Geometry check sheet. Reference: the model listing, model coordinates, mm. Give positions to 0.01 mm unless a question says otherwise; leave off trailing zeros. Order: outer loops, then holes, each group sorted by start corner. A loop starts at its lowest first (then second) coordinate and runs counter-clockwise, first axis right, second up.
from build123d import *

# Parameters (mm, degrees)
SKETCH1_R           = 1.355900406
BOSS_EXTRUDE1_DEPTH = 1.5875
SKETCH2_R           = 3.175
BOSS_EXTRUDE2_DEPTH = 1.5875
SKETCH3_R           = 1.524
CUT_EXTRUDE1_DEPTH  = 436.184338179
SKETCH5_W           = 2.10299656
SKETCH5_H           = 13.208
BOSS_EXTRUDE3_DEPTH = 1.5875


with BuildPart() as part:
    # Sketch1 → Boss-Extrude1 (new body)
    with BuildSketch(Plane.XY):
        with BuildLine():
            Line((-301.9473, 111.74645), (-305.87795, 115.6771))
            Line((-305.87795, 115.6771), (-316.1078, 115.6771))
            Line((-316.1078, 115.6771), (-316.1078, 128.8851))
            Line((-316.1078, 128.8851), (-305.87795, 128.8851))
            Line((-305.87795, 128.8851), (-301.9473, 132.81575))
            Line((-301.9473, 132.81575), (-301.9473, 150.9704))
            ThreePointArc((-301.9473, 150.9704), (-303.063223164, 153.664476836), (-305.7573, 154.7804))
            Line((-305.7573, 154.7804), (-397.247125, 154.7804))
            ThreePointArc((-397.247125, 154.7804), (-399.946077222, 153.659592612), (-401.0571, 150.956597849))
            Line((-401.0571, 150.956597849), (-401.0571, 148.341))
            Line((-401.0571, 148.341), (-399.1521, 148.341))
            Line((-399.1521, 148.341), (-399.1521, 95.6449))
            Line((-399.1521, 95.6449), (-401.0571, 95.6449))
            Line((-401.0571, 95.6449), (-401.0571, 91.659304166))
            ThreePointArc((-401.0571, 91.659304166), (-399.951018769, 88.947400452), (-397.2472, 87.8217))
            Line((-397.2472, 87.8217), (-378.5565, 87.8217))
            Line((-378.5565, 87.8217), (-368.3165, 91.1883))
            Line((-368.3165, 91.1883), (-315.9973, 91.1883))
            Line((-315.9973, 91.1883), (-305.7573, 87.8217))
            ThreePointArc((-305.7573, 87.8217), (-303.063223164, 88.937623164), (-301.9473, 91.6317))
            Line((-301.9473, 91.6317), (-301.9473, 111.74645))
        make_face()
        with Locations((-305.7573, 91.6317)):
            Circle(SKETCH1_R, mode=Mode.SUBTRACT)
        with Locations((-305.7573, 150.9704)):
            Circle(SKETCH1_R, mode=Mode.SUBTRACT)
        with Locations((-397.247125, 150.9704)):
            Circle(SKETCH1_R, mode=Mode.SUBTRACT)
        with Locations((-397.2472, 91.6317)):
            Circle(SKETCH1_R, mode=Mode.SUBTRACT)
    extrude(amount=BOSS_EXTRUDE1_DEPTH)

    # Sketch2 → Boss-Extrude2 (add)
    # profile 1 of 2: a face of its own
    with BuildSketch(Plane.XY.offset(1.5875)):
        with BuildLine():
            Line((-361.0272, 159.40105), (-361.0272, 154.7804))
            Line((-361.0272, 154.7804), (-341.9772, 154.7804))
            Line((-341.9772, 154.7804), (-341.9772, 159.40105))
            ThreePointArc((-341.9772, 159.40105), (-351.5022, 168.92605), (-361.0272, 159.40105))
        make_face()
        with Locations((-351.5022, 159.40105)):
            Circle(SKETCH2_R, mode=Mode.SUBTRACT)
    # profile 2 of 2: a face of its own
    with BuildSketch(Plane.XY.offset(1.5875)):
        with BuildLine():
            Line((-341.9772, 91.1883), (-361.0272, 91.1883))
            Line((-361.0272, 91.1883), (-361.0272, 83.20105))
            ThreePointArc((-361.0272, 83.20105), (-351.5022, 73.67605), (-341.9772, 83.20105))
            Line((-341.9772, 83.20105), (-341.9772, 91.1883))
        make_face()
        with Locations((-351.5022, 83.20105)):
            Circle(SKETCH2_R, mode=Mode.SUBTRACT)
    extrude(amount=-BOSS_EXTRUDE2_DEPTH)

    # Sketch3 → Cut-Extrude1 (cut, through all)
    with BuildSketch(Plane.XY.offset(1.5875)):
        with Locations((-397.247125, 150.9704)):
            Circle(SKETCH3_R)
        with Locations((-305.7573, 150.9704)):
            Circle(SKETCH3_R)
        with Locations((-305.7573, 91.6317)):
            Circle(SKETCH3_R)
        with Locations((-397.2472, 91.6317)):
            Circle(SKETCH3_R)
    extrude(amount=-CUT_EXTRUDE1_DEPTH, mode=Mode.SUBTRACT)

    # Sketch5 → Boss-Extrude3 (add)
    with BuildSketch(Plane.XY.offset(1.5875)):
        with Locations((-315.05630172, 122.2811)):
            Rectangle(SKETCH5_W, SKETCH5_H)
    extrude(amount=-BOSS_EXTRUDE3_DEPTH)


solid = part.part
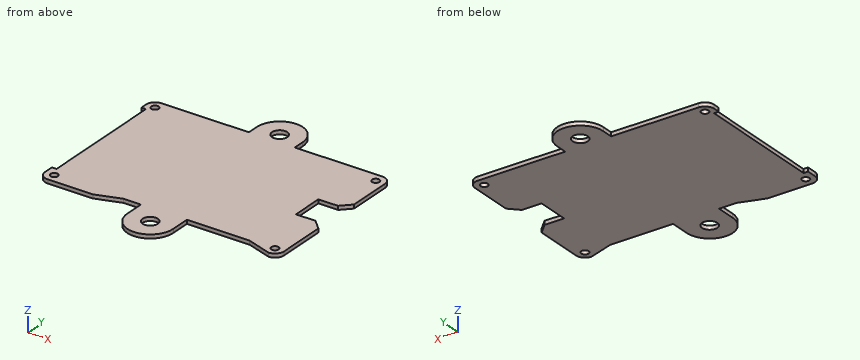
Item 1: Sectioned sample at D-D (y = 97.5). Enter the section's corners in (x, z), and give its area (3 significant figures).
Reported:
outline: (-399.15, 0) - (-301.95, 0) - (-301.95, 1.59) - (-399.15, 1.59) - close
area: 154 mm2
Item 2: Sectioned sample at B-B (z = 0.4). Give the number of separate pieces and of enclosed holes in the cut face, and give its area (3 significant figures).
Reported:
separate pieces: 1
enclosed holes: 6
area: 6,570 mm2
Item 3: Gauge pin test, flat ends, axial feed: pin 1 (0.5 mm diameter, centred on y = 86.5, z = 0.5, fed in from -X); pin 2 (4 mm diameter, centred on x = -397.25, y = 91.63, fed in from -Z); pin 3 (0.5 mm diameter, centred on x = -400.5, z = 0.5, fed in from +Y); pin 4 (0.8 mm diameter, centred on y = 120, z = 0.5, fed in from -X). Record the tip position at first contact, or that the pin passes through.
Reported:
pin 1: stops at x = -361.03
pin 2: stops at z = 0
pin 3: stops at y = 153.32
pin 4: stops at x = -399.15
Item 4: Sectioned sample at A-A (x = -350.5). Enter the section's corners in (y, z), and give its area (3 significant figures).
Reported:
outline: (73.73, 0) - (80.19, 0) - (80.19, 1.59) - (73.73, 1.59) - close; (86.21, 0) - (156.39, 0) - (156.39, 1.59) - (86.21, 1.59) - close; (162.41, 0) - (168.87, 0) - (168.87, 1.59) - (162.41, 1.59) - close
area: 132 mm2
Item 5: Sectioned sample at C-C (x = -327). Enter the section's corners in (y, z).
Reported:
outline: (91.19, 0) - (154.78, 0) - (154.78, 1.59) - (91.19, 1.59) - close
Item 6: Scan lines: L1, parallel to Y at x = -350, z = 0.6; L2, parallel to X at y = 151.5, z = 0.65; L3, parallel to X at y = 150.5, z = 0.25. Record each from-to range of solid material in increasing order.
Reported:
L1: y = 73.8 to 80.4, 86 to 156.6, 162.2 to 168.81
L2: x = -401.02 to -398.68, -395.82 to -307.19, -304.33 to -301.98
L3: x = -401.06 to -398.7, -395.8 to -307.21, -304.31 to -301.95
